For this review, take the finished solid that the model builds, in its own axes (mm). Round coordinates to 2 decimals unless told otherwise and drop trailing zeros. Write each loop counter-clockwise with the first axis right and the second up, starting at its lowest first coordinate (ties: lowest second). Pieces come first, ordered by that corner, then holes. Notation, with made-up numbers: (10.5, 29.25) -> (42.5, 29.25) arc R22 ccw to (42.5, 48.25) -> close; hole circle Ø9 at (-29.5, 61.25). An arc over 180 degrees is marked (long way). Answer in a Markdown table with one row per item.
from build123d import *

# Parameters (mm, degrees)
SKETCH1_R           = 4.1656
BOSS_EXTRUDE1_DEPTH = 6.35


with BuildPart() as part:
    # Sketch1 → Boss-Extrude1 (new body)
    with BuildSketch(Plane(origin=(0, 0, 0), x_dir=(1, 0, 0), z_dir=(0, 1, 0))):
        Polygon((-73.100424588, 81.91031941), (-35.000424588, 81.91031941), (3.099575412, 5.71031941), (3.099575412, -32.38968059), (-35.000424588, -108.58968059), (-73.100424588, -108.58968059), (-111.200424588, -32.38968059), (-111.200424588, 5.71031941), align=None)
        with Locations(Location((-92.150424588, -13.33968059, 0), (0, 0, 270))):
            Circle(SKETCH1_R, mode=Mode.SUBTRACT)
        with Locations(Location((-54.050424588, -13.33968059, 0), (0, 0, 270))):
            Circle(SKETCH1_R, mode=Mode.SUBTRACT)
        with Locations(Location((-15.950424588, -13.33968059, 0), (0, 0, 270))):
            Circle(SKETCH1_R, mode=Mode.SUBTRACT)
        with Locations(Location((-54.050424588, 24.76031941, 0), (0, 0, 270))):
            Circle(SKETCH1_R, mode=Mode.SUBTRACT)
        with Locations(Location((-54.050424588, 62.86031941, 0), (0, 0, 270))):
            Circle(SKETCH1_R, mode=Mode.SUBTRACT)
        with Locations(Location((-54.050424588, -51.43968059, 0), (0, 0, 270))):
            Circle(SKETCH1_R, mode=Mode.SUBTRACT)
        with Locations(Location((-54.050424588, -89.53968059, 0), (0, 0, 270))):
            Circle(SKETCH1_R, mode=Mode.SUBTRACT)
    extrude(amount=BOSS_EXTRUDE1_DEPTH)


solid = part.part
1) Consider section C-C on x = -7. State the section outline as (y, z) points.
Solved:
| item | result |
|---|---|
| outline | (0, -25.91) -> (6.35, -25.91) -> (6.35, 52.59) -> (0, 52.59) -> close |
2) Mouldability with a two-part tool opening along Z and no side actions: class faces 1 (the flat face through (-91.884, 3.131, 71.023)), 2 (the flat face through (3.1, 3, 13)), 3 (the cylindrical face through (-58.117, 3.131, -63.763)) as pulls with the +Z half, pulls with the -Z half, needs draft (parallel to the pull), parting line crosses it, or undercut.
Solved:
| item | result |
|---|---|
| face 1 | pulls with the +Z half |
| face 2 | needs draft |
| face 3 | undercut |
3) Consider section D-D on z = -42.5. State the section outline as (x, y) points, then the cut area to 3 significant figures.
Solved:
| item | result |
|---|---|
| outline | (-92.81, 0) -> (-15.3, 0) -> (-15.3, 6.35) -> (-92.81, 6.35) -> close |
| area | 492 mm² |
4) Consider section B-B on y = 4.5. State the section outline as (x, z) points.
Solved:
| item | result |
|---|---|
| outline | (-111.2, -5.71) -> (-73.1, -81.91) -> (-35, -81.91) -> (3.1, -5.71) -> (3.1, 32.39) -> (-35, 108.59) -> (-73.1, 108.59) -> (-111.2, 32.39) -> close; hole circle Ø8.33 at (-92.15, 13.34); hole circle Ø8.33 at (-54.05, -62.86); hole circle Ø8.33 at (-54.05, -24.76); hole circle Ø8.33 at (-54.05, 13.34); hole circle Ø8.33 at (-54.05, 51.44); hole circle Ø8.33 at (-54.05, 89.54); hole circle Ø8.33 at (-15.95, 13.34) |
5) For line 1 (X direction, y = 5.75, z = 54); line 2 (X direction, y = 5.5, z = -21.5); line 3 (X direction, y = 2.75, z = 10), list the stretches that pass through material, from the lowest coordinate up. Write a range as [from, to].
Solved:
| item | result |
|---|---|
| line 1 | [-100.4, -57.34], [-50.76, -7.71] |
| line 2 | [-103.31, -56.64], [-51.46, -4.8] |
| line 3 | [-111.2, -94.64], [-89.66, -56.54], [-51.56, -18.44], [-13.46, 3.1] |
6) Clearance check with a flat-ended pin moving along its axis: pin 1 Ø1.5 at (x, y) = (-97, 2) entering from +Z. State where the tip first meets the part, or that it passes through.
Solved:
| item | result |
|---|---|
| pin 1 | z = 62.29 |
7) Consider section A-A on z = 50. State the section outline as (x, y) points.
Solved:
| item | result |
|---|---|
| outline | (-102.4, 0) -> (-57.96, 0) -> (-57.96, 6.35) -> (-102.4, 6.35) -> close; (-50.14, 0) -> (-5.71, 0) -> (-5.71, 6.35) -> (-50.14, 6.35) -> close |
